For this review, take the finished solid that the model builds, in its own axes (mm). A direction names the side the tool comes from. Coordinates: 2 decimals unless noted, no trailing zeros. Write each loop counter-clockwise with the first axis right and the second up, starting at its lowest first coordinate (ties: lowest second). Pieces come first, ordered by that corner, then holes.
1) We need section B-B on y = 26.5. Write out the cut boundary in (x, z) (3 decimals), then the cut area to 3 significant figures.
2) Insertion check: P1, Ø23, axis at x = 45.5, z = 8, coming from the -Y side; P2, Ø6, axis at x = 58.5, y = 11.5, coming from the +Z side; P3, Ø10, axis at x = 16, y = 70.5, coming from the +Z side; P4, Ø1.5, axis at x = 33.5, y = 17, coming from the +Z side (3 decimals). Each pin has a flat end and moves straight along its axis. Give the tip position at first contact, or say it passes through.
3) We need section D-D on z = 43. Write out the cut boundary in (x, y), then the cut area to 3 significant figures.
4) To check wall thickness, follow line 1 along X through (y, z) = (72, -6); line 2 along Z through (x, y) = (58.9, 3.8); line 3 along Z through (x, y) = (33, 46). State the ranges of each line that lie inside material, in increasing order.
5) We need section A-A on z = -6.05. Write out the cut boundary in (x, y), then the cut area to 3 significant figures.
6) We need section C-C on x = 33.5. Write out the cut boundary in (y, z) (3 decimals).
7) Mouldability with a two-part tool opening along Y and no side actions: class faces 1 (the face through (7.412, 2.504, 12.624)), 2 (the face through (33, 5.08, 28)), 3 (the face through (12, 38.28, 44)) as pulls with the +Y half, pulls with the -Y half, needs draft (parallel to the pull), parting line crosses it, or undercut.
8) For faces 4 (the face through (53.67, 21.45, 43.6)), 5 (the face through (58, 70, -21)), 6 (the face through (54, 73, -11)), list the 3-axis set-ups (+Z, -Z, +X, -X, +Y, -Y) from which the entire face can be reached by the end or side of a thin tool; tool diameter is ignored.
from build123d import *

# Parameters (mm, degrees)
SKETCH1_W           = 67
SKETCH1_H           = 57.15
SKETCH1_R           = 3.175
BOSS_EXTRUDE1_DEPTH = 5.08
SKETCH2_R           = 27.67
SKETCH2_R_2         = 24.13
BOSS_EXTRUDE2_DEPTH = 76.2
BOSS_EXTRUDE3_REACH = 59.15
SKETCH4_W           = 55.34
SKETCH4_H           = 43
SKETCH5_W           = 7.17
SKETCH5_H           = 3.2
BOSS_EXTRUDE4_DEPTH = 21
SKETCH6_R           = 2.5
CUT_EXTRUDE1_DEPTH  = 11
SKETCH7_W           = 7.17
SKETCH7_H           = 3.2
BOSS_EXTRUDE5_DEPTH = 2
SKETCH8_W           = 7.17
SKETCH8_H           = 2
BOSS_EXTRUDE6_DEPTH = 3.2
SKETCH9_R           = 6.6
CUT_EXTRUDE2_DEPTH  = 33.2


with BuildPart() as part:
    # Sketch1 → Boss-Extrude1 (new body)
    with BuildSketch(Plane(origin=(0, 0, 0), x_dir=(1, 0, 0), z_dir=(0, 1, 0))):
        with Locations((33.5, -28.575)):
            Rectangle(SKETCH1_W, SKETCH1_H)
        with Locations((8.1, -9.525)):
            Circle(SKETCH1_R, mode=Mode.SUBTRACT)
        with Locations((58.9, -9.525)):
            Circle(SKETCH1_R, mode=Mode.SUBTRACT)
        with Locations((58.9, -47.625)):
            Circle(SKETCH1_R, mode=Mode.SUBTRACT)
        with Locations((8.1, -47.625)):
            Circle(SKETCH1_R, mode=Mode.SUBTRACT)
    extrude(amount=BOSS_EXTRUDE1_DEPTH)

    # Sketch2 → Boss-Extrude2 (add)
    with BuildSketch(Plane(origin=(0, 5.08, 0), x_dir=(1, 0, 0), z_dir=(0, 1, 0))):
        with Locations((33.5, -28.575)):
            Circle(SKETCH2_R)
        with Locations((33.5, -28.575)):
            Circle(SKETCH2_R_2, mode=Mode.SUBTRACT)
    extrude(amount=BOSS_EXTRUDE2_DEPTH)

    # Sketch4 → Boss-Extrude3 (add, up to next)
    with BuildSketch(Plane(origin=(0, 0, 0), x_dir=(-1, 0, 0), z_dir=(0, 0, -1)), mode=Mode.PRIVATE) as boss_extrude3_sk1:
        with Locations((-33.5, 59.78)):
            Rectangle(SKETCH4_W, SKETCH4_H)
    boss_extrude3_tool1 = extrude(boss_extrude3_sk1.sketch, amount=-BOSS_EXTRUDE3_REACH, mode=Mode.PRIVATE) - part.part
    add(boss_extrude3_tool1.solids().sort_by_distance((33.5, 59.78, 0))[0])

    # Sketch5 → Boss-Extrude4 (add)
    with BuildSketch(Plane(origin=(0, 0, 0), x_dir=(-1, 0, 0), z_dir=(0, 0, -1))):
        with Locations((-9.415, 72.88)):
            Rectangle(SKETCH5_W, SKETCH5_H)
        with Locations((-57.585, 72.88)):
            Rectangle(SKETCH5_W, SKETCH5_H)
    extrude(amount=BOSS_EXTRUDE4_DEPTH)

    # Sketch6 → Cut-Extrude1 (cut, through all)
    with BuildSketch(Plane.XZ.offset(-71.28)):
        with Locations((9.2, -6.05)):
            Circle(SKETCH6_R)
        with Locations((57.8, -6.05)):
            Circle(SKETCH6_R)
        with Locations((57.8, -14.95)):
            Circle(SKETCH6_R)
        with Locations((9.2, -14.95)):
            Circle(SKETCH6_R)
    extrude(amount=-CUT_EXTRUDE1_DEPTH, mode=Mode.SUBTRACT)

    # Sketch7 → Boss-Extrude5 (add)
    with BuildSketch(Plane(origin=(0, 0, -21), x_dir=(-1, 0, 0), z_dir=(0, 0, -1))):
        with Locations((-57.585, 72.88)):
            Rectangle(SKETCH7_W, SKETCH7_H)
        with Locations((-9.415, 72.88)):
            Rectangle(SKETCH7_W, SKETCH7_H)
    extrude(amount=BOSS_EXTRUDE5_DEPTH)

    # Sketch8 → Boss-Extrude6 (add)
    with BuildSketch(Plane.XZ.offset(-71.28)):
        with Locations((9.415, -22)):
            Rectangle(SKETCH8_W, SKETCH8_H)
        with Locations((57.585, -22)):
            Rectangle(SKETCH8_W, SKETCH8_H)
    extrude(amount=BOSS_EXTRUDE6_DEPTH)

    # Sketch9 → Cut-Extrude2 (cut)
    with BuildSketch(Plane(origin=(0, 5.08, 0), x_dir=(1, 0, 0), z_dir=(0, 1, 0))):
        with Locations((8.1, -9.525)):
            Circle(SKETCH9_R)
        with Locations((58.9, -9.525)):
            Circle(SKETCH9_R)
        with Locations((58.9, -47.625)):
            Circle(SKETCH9_R)
        with Locations((8.1, -47.625)):
            Circle(SKETCH9_R)
    extrude(amount=CUT_EXTRUDE2_DEPTH, mode=Mode.SUBTRACT)


solid = part.part
Result:
1. outline: (8.808, 16.087) arc R6.6 cw to (14.598, 8.368) arc R27.67 ccw to (52.402, 8.368) arc R6.6 cw to (58.192, 16.087) arc R27.67 ccw to (58.192, 41.063) arc R6.6 cw to (52.402, 48.782) arc R27.67 ccw to (14.598, 48.782) arc R6.6 cw to (8.808, 41.063) arc R27.67 ccw to start; hole circle Ø48.26 at (33.5, 28.575)
1. area: 509 mm2
2. P1: stops at y = 0
2. P2: stops at z = 41.97
2. P3: stops at z = 53.26
2. P4: stops at z = 56.245
3. outline: (0, 0) - (67, 0) - (67, 5.08) - (54.19, 5.08) - (54.19, 38.28) - (57.11, 38.28) - (57.11, 81.28) - (52.84, 81.28) - (52.84, 5.08) - (14.16, 5.08) - (14.16, 81.28) - (9.89, 81.28) - (9.89, 38.28) - (12.81, 38.28) - (12.81, 5.08) - (0, 5.08) - close
3. area: 797 mm2
4. line 1: x = 5.83 to 6.7, 11.7 to 13, 54 to 55.3, 60.3 to 61.17
4. line 2: z = 0 to 6.35, 12.7 to 44.45, 50.8 to 57.15
4. line 3: z = 0 to 4.45, 52.7 to 56.24
5. outline: (5.83, 71.28) - (6.7, 71.28) - (6.7, 74.48) - (5.83, 74.48) - close; (11.7, 71.28) - (13, 71.28) - (13, 74.48) - (11.7, 74.48) - close; (54, 71.28) - (55.3, 71.28) - (55.3, 74.48) - (54, 74.48) - close; (60.3, 71.28) - (61.17, 71.28) - (61.17, 74.48) - (60.3, 74.48) - close
5. area: 13.9 mm2
6. outline: (0, 0) - (5.08, 0) - (5.08, 0.905) - (38.28, 0.905) - (38.28, 0) - (81.28, 0) - (81.28, 4.445) - (5.08, 4.445) - (5.08, 52.705) - (81.28, 52.705) - (81.28, 56.245) - (5.08, 56.245) - (5.08, 57.15) - (0, 57.15) - close
7. face 1: needs draft
7. face 2: pulls with the +Y half
7. face 3: undercut
8. face 4: +X
8. face 5: +X, -X, -Y
8. face 6: -Z, +Y, -Y
